The model under review builds one solid part; all positions refer to its coordinate system, in mm. Face numbers are marked on the shaded views. A direction names the side the tool comes from. Round coordinates to 2 decimals unless told otherwise and drop trailing zeros. Order: outer loops, then holes, each group sorted by start corner. A loop starts at its lowest first (then second) coordinate and runs counter-clockwise, first axis right, second up. Notation, with made-up numbers: M 27.25,62 L 65.25,62 A24 ccw 65.25,100 Z; hole C 22,46.25 d10. An arc over 180 degrees is marked long. One line per item, written item: value. Start each with the question number.
Autodesk Inventor part; units mm, degrees
ref_plane "YZ Plane" through (0, 0, 0) normal (1, 0, 0) x (0, 1, 0)
ref_plane "XZ Plane" through (0, 0, 0) normal (0, 1, 0) x (-1, 0, 0)
ref_plane "XY Plane" through (0, 0, 0) normal (0, 0, 1) x (1, 0, 0)
sketch "Skizze1" plane through (0, 0, 0) normal (0, 0, 1) x (1, 0, 0)
  line L0 (0, 0) -> (127.5, 0)
  line L1 (127.5, 0) -> (127.5, -85.5)
  line L2 (127.5, -85.5) -> (0, -85.5)
  line L3 (0, -85.5) -> (0, 0)
  dimension "d0" = 127.5
  dimension "d1" = 85.5
extrude "Extrusion1" add sketch "Skizze1" along normal blind 5
sketch "Skizze2" plane through (0, 0, 5) normal (0, 0, 1) x (1, 0, 0)
  line L0 (0, -16.25) -> (3, -16.25)
  line L1 (3, -16.25) -> (3, -69.25)
  line L2 (3, -69.25) -> (0, -69.25)
  line L3 (0, -69.25) -> (0, -16.25)
  line L4 (63.75, 42.9175) -> (63.75, -147.2432)
  line L5 (127.5, -85.5) -> (127.5, 0)
  line L6 (127.5, -16.25) -> (124.5, -16.25)
  line L7 (124.5, -16.25) -> (124.5, -69.25)
  line L8 (124.5, -69.25) -> (127.5, -69.25)
  line L9 (127.5, -69.25) -> (127.5, -16.25)
  point P0 (0, 0)
  dimension "d4" = 3
  dimension "d5" = 53
  dimension "d6" = 16.25
  dimension "d7" = 63.75
extrude "Extrusion2" add sketch "Skizze2" along normal blind 7
fillet "Rundung1" radius 2 4 edges at (0, 0, 2.5) (127.5, 0, 2.5) (127.5, -85.5, 2.5) (0, -85.5, 2.5)
fillet "Rundung2" radius 1.5 8 edges at (3, -69.25, 8.5) (0, -69.25, 8.5) (3, -16.25, 8.5) (0, -16.25, 8.5) (124.5, -16.25, 8.5) (127.5, -16.25, 8.5) (124.5, -69.25, 8.5) (127.5, -69.25, 8.5)
sketch "Skizze3" plane through (0, 0, 5) normal (0, 0, 1) x (1, 0, 0)
  circle A0 centre (63.75, -42.75) radius 17.5
  line L0 (0, -67.75) -> (0, -83.5)
  point P0 (0, 0)
  dimension "d12" = 35
  dimension "d13" = 63.75
  dimension "d14" = 42.75
extrude "Extrusion3" cut sketch "Skizze3" against normal blind 10
hole "Bohrung1" at (63.75, -42.75, 5) direction (0, 0, -1) diameter 38.3 depth 3
sketch "Skizze4" plane through (0, 0, 0) normal (0, 0, -1) x (-1, 0, 0)
  line L0 (-125.5, -85.5) -> (-2, -85.5)
  line L1 (0, -83.5) -> (0, -2)
  line L2 (-12, -77.75) -> (-50.2871, -77.75)
  line L3 (-50.2871, -7.75) -> (-12, -7.75)
  line L4 (-12, -7.75) -> (-12, -77.75)
  line L5 (-63.75, -42.75) -> (-63.75, -99.3052)
  line L6 (-115.5, -77.75) -> (-77.2129, -77.75)
  line L7 (-77.2129, -7.75) -> (-115.5, -7.75)
  line L8 (-115.5, -7.75) -> (-115.5, -77.75)
  arc A0 (-50.2871, -77.75) -> (-50.2871, -7.75) centre (-63.75, -42.75) ccw
  arc A1 (-77.2129, -7.75) -> (-77.2129, -77.75) centre (-63.75, -42.75) ccw
  arc A2 (-50.2871, -77.75) -> (-50.2871, -7.75) centre (-63.75, -42.75) ccw
  arc A3 (-77.2129, -7.75) -> (-77.2129, -77.75) centre (-63.75, -42.75) ccw
  point P0 (0, 0)
  dimension "d27" = 42.75
  dimension "d28" = 63.75
  dimension "d29" = 12
  dimension "d30" = 70
  dimension "d31" = 7.75
extrude "Extrusion4" cut sketch "Skizze4" against normal blind 10
fillet "Rundung3" radius 7 4 edges at (50.2871, -77.75, 2.5) (77.2129, -77.75, 2.5) (50.2871, -7.75, 2.5) (77.2129, -7.75, 2.5)
fillet "Rundung4" radius 7 4 edges at (12, -77.75, 2.5) (115.5, -77.75, 2.5) (12, -7.75, 2.5) (115.5, -7.75, 2.5)
sketch "Skizze5" plane through (0, 0, 5) normal (0, 0, 1) x (1, 0, 0)
  circle A0 centre (63.75, -42.75) radius 19.15
  circle A1 centre (63.75, -42.75) radius 26
  line L0 (125.5, 0) -> (2, 0)
  point P0 (0, 0)
  dimension "d36" = 38.3
  dimension "d37" = 52
  dimension "d38" = 42.75
  dimension "d39" = 63.75
extrude "Extrusion5" add sketch "Skizze5" along normal blind 7
sketch "Skizze6" plane through (63.75, -42.75, 12) normal (0, 0, 1) x (1, 0, 0)
  circle A0 centre (0, 22.5) radius 2.525
  circle A1 centre (0, 0) radius 17.5
  point P0 (-63.75, 42.75)
  dimension "d44" = 5.05
  dimension "d45" = 22.5
extrude "Extrusion6" cut sketch "Skizze6" against normal blind 2.1 contours A0
pattern_circular "Runde Anordnung1" count 3 over 360 about axis through (63.75, -42.75, 5) along (0, 0, 1) of "Extrusion6"
properties part number "Sensor Halterung381"
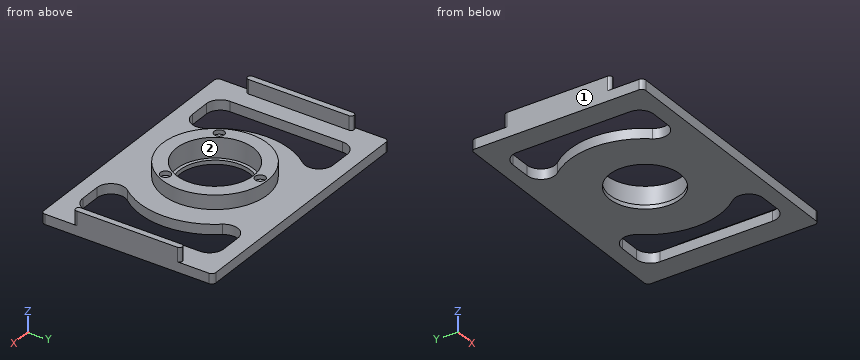
Item 1: Clearance check with flat-ended pins moving along their axes: P1, Ø4, axis at y = -20, z = 7, coming from the -X side; P2, Ø11.5, axis at x = 56.5, y = -37.5, coming from the +Z side; P3, Ø4, axis at x = 63.75, y = -20.25, coming from the +Z side; P4, Ø2, axis at x = 82.5, y = -16, coming from the +Z side. State where each tip first meets the part, or that it passes through.
Item 2: Consider section D-D, the plane y = -12. Give the boundary of the cut face in (x, z), then the cut area to 3 significant figures.
Item 3: Consider section B-B, the plane y = -33. Give the boundary of the cut face in (x, z), then the cut area to 3 significant figures.
Item 4: Machinability: for the marked faces 1 and 2, which of the approach directions +Z, -Z, +X, -X, +Y, -Y give a long, thin tool a straight path to every point of the face, cutting with its end or side? Answer none if there is none.
Item 5: Wall thickness on L1, parallel to X at y = -41, z = 8; L2, parallel to X at y = -20.5, z = 7.5; L3, parallel to X at y = -67, z = 4.75: over which ranges is each line inside the solid? List them lowest first.
Computed:
1. P1: stops at x = 0
1. P2: passes through
1. P3: stops at z = 9.9
1. P4: stops at z = 5
2. outline: M 0,0 L 12.56,0 L 12.56,5 L 0,5 Z; M 35.6,0 L 91.9,0 L 91.9,5 L 35.6,5 Z; M 114.94,0 L 127.5,0 L 127.5,5 L 114.94,5 Z
2. area: 407 mm^2
3. outline: M 0,0 L 12,0 L 12,5 L 3,5 L 3,12 L 0,12 Z; M 27.54,0 L 49.22,0 L 49.22,2 L 47.27,2 L 47.27,12 L 39.65,12 L 39.65,5 L 27.54,5 Z; M 78.28,0 L 99.96,0 L 99.96,5 L 87.85,5 L 87.85,12 L 80.23,12 L 80.23,2 L 78.28,2 Z; M 115.5,0 L 127.5,0 L 127.5,12 L 124.5,12 L 124.5,5 L 115.5,5 Z
3. area: 474 mm^2
4. face 1: +Z, -Z, -X, +Y, -Y
4. face 2: +Z
5. L1: x = 0 to 3, 37.81 to 44.68, 82.82 to 89.69, 124.5 to 127.5
5. L2: x = 0 to 3, 50.3 to 77.2, 124.5 to 127.5
5. L3: x = 0 to 12, 35.07 to 92.43, 115.5 to 127.5
